The listing builds one solid part. Answer for the finished solid, in the listing's coordinates (mm). Give positions to 0.01 mm unless a question says otherwise; leave off trailing zeros. Write each loop counter-clockwise with the first axis right and the second up, starting at its lowest first coordinate (ties: lowest second). Pieces come first, ordered by that corner, then holes. Notation, with made-up numbers: (21.25, -7.75) - (30.25, -7.75) arc R27 ccw to (30.25, 19.25) - close; hole circle Ø4 at (55, 8). An arc over 180 degrees is marked (long way). Answer as CSV lines item,"result". Start each with the question number.
(1) Each of these flat-tipped pins is pushed along its axis until it touches: pin 1 Ø1.6 at (y, z) = (1478.5, 2) entering from +X; pin 2 Ø10 at (x, y) = (-1024.5, 1474) entering from +Z (3 decimals); pin 3 Ø14 at (x, y) = (-1031.59, 1466.99) entering from +Z. Where does it stop, or does it pass through?
(2) Find section B-B (x = -975). Write down the section's boundary in (y, z) (3 decimals).
(3) Find section A-A (y = 1461.5). Write down the section's boundary in (x, z) (3 decimals), then the cut area to 3 significant figures.
(4) Straight lines are drawn through the part: probe 1 along Y at (x, z) = (-1016, 1.4); probe 2 along X at (y, z) = (1481.5, 1.7); probe 3 along Y at (x, z) = (-1048, 0.75). For each, find the intervals that lie inside material, in ascending order.
(5) Find section C-C (z = 2.3). State how many separate pieces and enclosed holes the cut face has, then the cut area to 3 significant figures.
(6) Find section D-D (y = 1468.5). Write down the section's boundary in (x, z) (3 decimals), then the cut area to 3 significant figures.
from build123d import *

# Parameters (mm, degrees)
BOSS_EXTRUDE1_DEPTH = 3.175
SKETCH3_R           = 11.8
SKETCH3_R_2         = 1.8
CUT_EXTRUDE1_DEPTH  = 1823.683867823
SKETCH4_R           = 3.15
CUT_EXTRUDE2_DEPTH  = 1823.683867823


with BuildPart() as part:
    # Sketch1 → Boss-Extrude1 (new body)
    with BuildSketch(Plane.XY):
        Polygon((-1010.58632196, 1449.028372115), (-1010.58632196, 1458.511234066), (-944.581241408, 1458.511234066), (-944.581241408, 1475.511234066), (-1010.58632196, 1475.511234066), (-1010.58632196, 1485.028372115), (-1013.58632196, 1488.028372115), (-1049.58632196, 1488.028372115), (-1052.58632196, 1485.028372115), (-1052.58632196, 1449.028372115), (-1049.58632196, 1446.028372115), (-1013.58632196, 1446.028372115), align=None)
    extrude(amount=BOSS_EXTRUDE1_DEPTH)

    # Sketch3 → Cut-Extrude1 (cut, through all)
    with BuildSketch(Plane(origin=(0, 0, 0), x_dir=(-1, 0, 0), z_dir=(0, 0, -1))):
        with Locations((1031.58632196, 1466.994096018)):
            Circle(SKETCH3_R)
        with Locations((1047.08632196, 1482.494096018)):
            Circle(SKETCH3_R_2)
        with Locations((1047.08632196, 1451.494096018)):
            Circle(SKETCH3_R_2)
        with Locations((1016.08632196, 1451.494096018)):
            Circle(SKETCH3_R_2)
        with Locations((1016.08632196, 1482.494096018)):
            Circle(SKETCH3_R_2)
    extrude(amount=-CUT_EXTRUDE1_DEPTH, mode=Mode.SUBTRACT)

    # Sketch4 → Cut-Extrude2 (cut, through all)
    with BuildSketch(Plane.XY.offset(3.175)):
        with Locations((-973.927184785, 1466.986205253)):
            Circle(SKETCH4_R)
        with Locations((-993.918310147, 1466.990315025)):
            Circle(SKETCH4_R)
        with Locations((-954.241393614, 1466.990315025)):
            Circle(SKETCH4_R)
    extrude(amount=-CUT_EXTRUDE2_DEPTH, mode=Mode.SUBTRACT)


solid = part.part
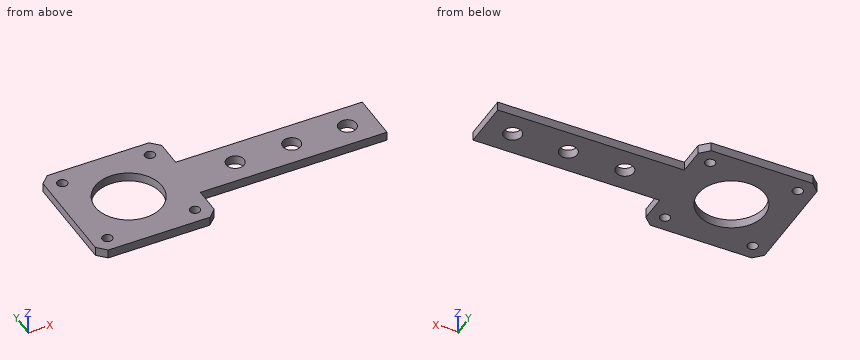
Result set:
1,pin 1,"x = -1010.59"
1,pin 2,"z = 3.175"
1,pin 3,"through"
2,outline,"(1458.511, 0) - (1464.025, 0) - (1464.025, 3.175) - (1458.511, 3.175) - close; (1469.948, 0) - (1475.511, 0) - (1475.511, 3.175) - (1469.948, 3.175) - close"
3,outline,"(-1052.586, 0) - (-1042.029, 0) - (-1042.029, 3.175) - (-1052.586, 3.175) - close; (-1021.143, 0) - (-944.581, 0) - (-944.581, 3.175) - (-1021.143, 3.175) - close"
3,area,"277 mm^2"
4,probe 1,"1446.03 to 1449.7, 1453.29 to 1480.7, 1484.29 to 1488.03"
4,probe 2,"-1052.59 to -1048.59, -1045.59 to -1017.59, -1014.59 to -1010.59"
4,probe 3,"1446.03 to 1449.94, 1453.04 to 1480.94, 1484.04 to 1488.03"
5,separate pieces,"1"
5,enclosed holes,"8"
5,area,"2,300 mm^2"
6,outline,"(-1052.586, 0) - (-1043.29, 0) - (-1043.29, 3.175) - (-1052.586, 3.175) - close; (-1019.883, 0) - (-996.683, 0) - (-996.683, 3.175) - (-1019.883, 3.175) - close; (-991.154, 0) - (-976.69, 0) - (-976.69, 3.175) - (-991.154, 3.175) - close; (-971.165, 0) - (-957.006, 0) - (-957.006, 3.175) - (-971.165, 3.175) - close; (-951.477, 0) - (-944.581, 0) - (-944.581, 3.175) - (-951.477, 3.175) - close"
6,area,"216 mm^2"
